Design review of the part built by this model. Coordinates are the model's own, in mm. A direction names the side the tool comes from. Give positions to 0.01 mm unless a question says otherwise; leave off trailing zeros. Loops run counter-clockwise (first coordinate to the right, second up) from the corner with the lowest first, then second, coordinate; pieces in that order, holes last. Notation, with made-up numbers: (42.5, -24.75) -> (75.5, -24.75) arc R22 cw to (75.5, -8.75) -> close; hole circle Ø5 at (-25, 84.25). An arc over 180 degrees is marked (long way). Answer in a Markdown table with one row per item. Add a question column.
(1) Draft analysis for pull direction X (two halves, no side actions). For faces 1 (the flat face through (81.026, 5, 0)), 2 (the cylindrical face through (0.771, 1.355, -0.068)), 3 (the flat face through (-5, 9.652, 0)), state which applies: +X half, -X half, draft (parallel to the pull), parting line (faces both ways), or undercut.
(2) For faces 4 (the cylindrical face through (42.393, 9.785, 1.101)), 5 (the flat face through (-7, 5, -4.826)), 6 (the flat face through (-5, 0, 0)), 7 (the flat face through (4.826, 1, -4)), 8 (the flat face through (4.826, 9, 4)), list the 3-axis set-ups (+Z, -Z, +X, -X, +Y, -Y) from which the entire face can be reached by the end or side of a thin tool; tool diameter is ignored.
(3) Consider section C-C on x = 46. Write out the cut boundary in (y, z).
(4) For pin 1 (5 mm diameter, centred on x = -11.5, y = 7, fed in from -Z); pin 2 (5.5 mm diameter, centred on x = 0, y = 4.826, fed in from -Z); pin 3 (5 mm diameter, centred on x = -11.5, z = 0.5, fed in from +Y); pin 4 (5 mm diameter, centred on x = -5, y = 5.5, fed in from +Z), all flat-tipped, find the tip position at first contact; note any pin that passes through.
(5) Consider section A-A on z = 0. Write out the cut boundary in (x, y).
(6) For line 1 (Y direction, x = 0, z = 4); line 2 (X direction, y = 7, z = 0); line 3 (X direction, y = 5.5, z = 2), list the stretches that pass through material, from the lowest coordinate up.
(7) Consider section B-B on x = -15.24. Write out the cut boundary in (y, z), then the cut area to 3 significant figures.
Autodesk Inventor part; units mm, degrees
ref_plane "YZ Plane" through (0, 0, 0) normal (1, 0, 0) x (0, 1, 0)
ref_plane "XZ Plane" through (0, 0, 0) normal (0, 1, 0) x (-1, 0, 0)
ref_plane "XY Plane" through (0, 0, 0) normal (0, 0, 1) x (1, 0, 0)
sketch "Sketch1" plane through (0, 0, 0) normal (0, 1, 0) x (-1, 0, 0)
  line L0 (0, 0) -> (15.24, 0)
  circle A0 centre (15.24, 0) radius 3.556
  circle A1 centre (0, 0) radius 3.556
  line L1 (18.796, 0) -> (20.066, 0)
  line L2 (15.24, -3.556) -> (15.24, -4.826)
  line L3 (15.24, -4.826) -> (0, -4.826)
  line L4 (-3.556, 0) -> (-4.826, 0)
  line L5 (-4.826, 0) -> (-4.826, -4.826)
  line L6 (-4.826, -4.826) -> (0, -4.826)
  line L7 (15.24, -4.826) -> (20.066, -4.826)
  line L8 (20.066, -4.826) -> (20.066, 0)
  line L9 (15.24, 3.556) -> (15.24, 4.826)
  line L10 (15.24, 4.826) -> (20.066, 4.826)
  line L11 (20.066, 4.826) -> (-4.826, 4.826)
  line L12 (-4.826, 4.826) -> (-4.826, 0)
  line L13 (0, -4.826) -> (-4.826, -4.826)
  line L14 (20.066, 4.826) -> (20.066, 0)
  dimension "d2" = 7.112
  dimension "d0" = 15.24
  dimension "d1" = 7.112
  dimension "d3" = 1.27
  dimension "d4" = 1.27
  dimension "d5" = 1.27
  dimension "d6" = 1.27
extrude "Extrusion1" add sketch "Sketch1" along normal blind 9.652 contours A1 L4 L12 L11 L9 A0 L0 | A1 | L0 A0 L2 L3 L6 L5 L4 A1 | L9 L10 L14 L1 A0 | A0 L1 L8 L7 L2
sketch "Sketch2" plane through (4.826, 0, -4.826) normal (0, 0, -1) x (-1, 0, 0)
  line L0 (0, 0) -> (0, 9.652)
  line L1 (0, 4.826) -> (4.826, 4.826)
  circle A0 centre (4.826, 4.826) radius 3.556
  point P0 (4.826, 0)
  dimension "d9" = 4.826
  dimension "d10" = 7.112
extrude "Extrusion2" cut sketch "Sketch2" against normal through all
sketch "Sketch3" plane through (4.826, 0, 4.826) normal (1, 0, 0) x (0, 0, -1)
  line L0 (4.826, 0) -> (4.826, 9.652)
  line L1 (0, 9.652) -> (9.652, 9.652)
  line L2 (0, 0) -> (0, 9.652)
  line L3 (0, 4.826) -> (9.652, 4.826)
  line L4 (9.652, 0) -> (9.652, 9.652)
  circle A0 centre (4.826, 4.826) radius 5.08
  dimension "d13" = 10.16
extrude "Extrusion3" add sketch "Sketch3" along normal blind 76.2 contours L3 L2 A0 L1 L0 | L3 L4 A0 L2 | L0 L1 A0 L4 L3 | L1 A0 | L2 A0 | L4 A0
sketch "Sketch4" plane through (81.026, 4.826, 0) normal (1, 0, 0) x (0, 0, -1)
  circle A0 centre (0, 0) radius 5.08
  point P0 (0, -4.826)
extrude "Extrusion4" cut sketch "Sketch4" against normal blind 76.2
sketch "Sketch5" plane through (4.826, 0, 4.826) normal (1, 0, 0) x (0, 0, -1)
  line L0 (9.652, 9.652) -> (0, 9.652)
  line L1 (4.826, 9.652) -> (4.826, 0)
  circle A0 centre (4.826, 4.826) radius 5.08
  dimension "d18" = 10.16
extrude "Extrusion5" add sketch "Sketch5" along normal blind 76.2
properties part number "newblock"
Values follow:
| question | item | result |
|---|---|---|
| 1 | face 1 | +X half |
| 1 | face 2 | undercut |
| 1 | face 3 | draft |
| 2 | face 4 | +X |
| 2 | face 5 | -Z, -X, +Y, -Y |
| 2 | face 6 | +Z, -Z, -X, -Y |
| 2 | face 7 | -Z, +X, -Y |
| 2 | face 8 | +Z, +X, +Y |
| 3 | outline | circle Ø10.16 at (4.83, 0) |
| 4 | pin 1 | z = -4.83 |
| 4 | pin 2 | through |
| 4 | pin 3 | y = 9.65 |
| 4 | pin 4 | z = 4.83 |
| 5 | outline | (-20.07, 0) -> (-18.8, 0) -> (-18.8, 9.65) -> (-20.07, 9.65) -> close; (-11.68, 0) -> (4.83, 0) -> (4.83, -0.25) -> (81.03, -0.25) -> (81.03, 9.91) -> (4.83, 9.91) -> (4.83, 9.65) -> (-11.68, 9.65) -> close; hole circle Ø7.11 at (0, 4.83) |
| 6 | line 1 | 0 to 1.27, 8.38 to 9.65 |
| 6 | line 2 | -20.07 to -18.8, -11.68 to -2.81, 2.81 to 81.03 |
| 6 | line 3 | -20.07 to -18.18, -12.3 to -3.49, 3.49 to 81.03 |
| 7 | outline | (0, -4.83) -> (9.65, -4.83) -> (9.65, -3.56) -> (0, -3.56) -> close; (0, 3.56) -> (9.65, 3.56) -> (9.65, 4.83) -> (0, 4.83) -> close |
| 7 | area | 24.5 mm2 |
